Could you check a few things on this model? Use its own coordinates, in mm. Face numbers are marked on the shaded views. Coordinates: 2 decimals unless noted, no trailing zeros. Write each loop counter-clockwise with the first axis right and the second up, starting at its lowest first coordinate (ties: lowest second). Pieces come first, ordered by that corner, then holes. Notation, with made-up numbers: (-37.5, -33.5) - (-21.5, -33.5) arc R11 ccw to (-21.5, -22.5) - close; hole circle Ø4 at (76, 39). An arc over 180 degrees is marked (long way). Write item = value, one per line. Start each with the question number.
```python
from build123d import *

# Parameters (mm, degrees)
SKETCH1_R           = 4.064
SKETCH1_R_2         = 2.794
BOSS_EXTRUDE1_DEPTH = 3.302
SKETCH2_R           = 0.62500002
BOSS_EXTRUDE2_DEPTH = 1.87000007
SKETCH4_R           = 1.449999894
CUT_EXTRUDE1_DEPTH  = 21.9977138
SKETCH5_R           = 3.555000002
SKETCH5_R_2         = 2.819999948
BOSS_EXTRUDE3_DEPTH = 0.470000076


with BuildPart() as part:
    # Sketch1 → Boss-Extrude1 (new body)
    with BuildSketch(Plane(origin=(0, 0, 0), x_dir=(1, 0, 0), z_dir=(0, 1, 0))):
        with Locations(Location((0, 0, 0), (0, 0, 90))):
            Circle(SKETCH1_R)
        with Locations(Location((0, 0, 0), (0, 0, 90))):
            Circle(SKETCH1_R_2, mode=Mode.SUBTRACT)
    extrude(amount=BOSS_EXTRUDE1_DEPTH)

    # Sketch2 → Boss-Extrude2 (add)
    with BuildSketch(Plane(origin=(0, 3.302, 0), x_dir=(1, 0, 0), z_dir=(0, 1, 0))):
        with BuildLine():
            Line((3.184398134, 6.598095019), (1.973411671, 13.950499548))
            ThreePointArc((1.973411671, 13.950499548), (0, 15.24), (-1.973411671, 13.950499548))
            Line((-1.973411671, 13.950499548), (-3.184398134, 6.598095019))
            ThreePointArc((-3.184398134, 6.598095019), (-3.525092211, 6.105638812), (-4.121918835, 6.05681719))
            Line((-4.121918835, 6.05681719), (-11.094781168, 8.684274414))
            ThreePointArc((-11.094781168, 8.684274414), (-13.198227153, 7.620000001), (-13.068192838, 5.266225136))
            Line((-13.068192838, 5.266225136), (-7.306316969, 0.54127783))
            ThreePointArc((-7.306316969, 0.54127783), (-7.050184422, 1e-09), (-7.306316969, -0.541277828))
            Line((-7.306316969, -0.541277828), (-13.068192838, -5.266225133))
            ThreePointArc((-13.068192838, -5.266225133), (-13.198227153, -7.619999998), (-11.094781167, -8.684274411))
            Line((-11.094781167, -8.684274411), (-4.121918835, -6.056817187))
            ThreePointArc((-4.121918835, -6.056817187), (-3.525092211, -6.10563881), (-3.184398134, -6.598095016))
            Line((-3.184398134, -6.598095016), (-1.973411671, -13.950499545))
            ThreePointArc((-1.973411671, -13.950499545), (0, -15.239999997), (1.973411671, -13.950499545))
            Line((1.973411671, -13.950499545), (3.184398134, -6.598095017))
            ThreePointArc((3.184398134, -6.598095017), (3.525092211, -6.10563881), (4.121918835, -6.056817187))
            Line((4.121918835, -6.056817187), (11.094781168, -8.684274411))
            ThreePointArc((11.094781168, -8.684274411), (13.198227153, -7.619999998), (13.068192838, -5.266225133))
            Line((13.068192838, -5.266225133), (7.306316969, -0.541277828))
            ThreePointArc((7.306316969, -0.541277828), (7.050184422, 1e-09), (7.306316969, 0.54127783))
            Line((7.306316969, 0.54127783), (13.068192838, 5.266225136))
            ThreePointArc((13.068192838, 5.266225136), (13.198227153, 7.620000001), (11.094781167, 8.684274413))
            Line((11.094781167, 8.684274413), (4.121918835, 6.05681719))
            ThreePointArc((4.121918835, 6.05681719), (3.525092211, 6.105638812), (3.184398134, 6.598095019))
        make_face()
        with Locations(Location((0, -7.50046633, 0), (0, 0, 270))):
            Circle(SKETCH2_R, mode=Mode.SUBTRACT)
        with Locations(Location((0, -10.500466426, 0), (0, 0, 270))):
            Circle(SKETCH2_R, mode=Mode.SUBTRACT)
        with Locations(Location((0, -13.500466522, 0), (0, 0, 270))):
            Circle(SKETCH2_R, mode=Mode.SUBTRACT)
        with Locations(Location((-11.691746971, -6.750233261, 0), (0, 0, 270))):
            Circle(SKETCH2_R, mode=Mode.SUBTRACT)
        with Locations(Location((-9.093670677, -5.250233213, 0), (0, 0, 270))):
            Circle(SKETCH2_R, mode=Mode.SUBTRACT)
        with Locations(Location((-6.495594382, -3.750233165, 0), (0, 0, 270))):
            Circle(SKETCH2_R, mode=Mode.SUBTRACT)
        with Locations(Location((-11.691746971, 6.750233261, 0), (0, 0, 270))):
            Circle(SKETCH2_R, mode=Mode.SUBTRACT)
        with Locations(Location((-9.093670677, 5.250233213, 0), (0, 0, 270))):
            Circle(SKETCH2_R, mode=Mode.SUBTRACT)
        with Locations(Location((-6.495594382, 3.750233165, 0), (0, 0, 270))):
            Circle(SKETCH2_R, mode=Mode.SUBTRACT)
        with Locations(Location((0, 13.500466522, 0), (0, 0, 270))):
            Circle(SKETCH2_R, mode=Mode.SUBTRACT)
        with Locations(Location((0, 10.500466426, 0), (0, 0, 270))):
            Circle(SKETCH2_R, mode=Mode.SUBTRACT)
        with Locations(Location((0, 7.50046633, 0), (0, 0, 270))):
            Circle(SKETCH2_R, mode=Mode.SUBTRACT)
        with Locations(Location((11.691746971, 6.750233261, 0), (0, 0, 270))):
            Circle(SKETCH2_R, mode=Mode.SUBTRACT)
        with Locations(Location((9.093670677, 5.250233213, 0), (0, 0, 270))):
            Circle(SKETCH2_R, mode=Mode.SUBTRACT)
        with Locations(Location((6.495594382, 3.750233165, 0), (0, 0, 270))):
            Circle(SKETCH2_R, mode=Mode.SUBTRACT)
        with Locations(Location((11.691746971, -6.750233261, 0), (0, 0, 270))):
            Circle(SKETCH2_R, mode=Mode.SUBTRACT)
        with Locations(Location((9.093670677, -5.250233213, 0), (0, 0, 270))):
            Circle(SKETCH2_R, mode=Mode.SUBTRACT)
        with Locations(Location((6.495594382, -3.750233165, 0), (0, 0, 270))):
            Circle(SKETCH2_R, mode=Mode.SUBTRACT)
    extrude(amount=BOSS_EXTRUDE2_DEPTH)

    # Sketch4 → Cut-Extrude1 (cut, through all)
    with BuildSketch(Plane(origin=(0, 5.17200007, 0), x_dir=(1, 0, 0), z_dir=(0, 1, 0))):
        with Locations(Location((0, 0, 0), (0, 0, 270))):
            Circle(SKETCH4_R)
    extrude(amount=-CUT_EXTRUDE1_DEPTH, mode=Mode.SUBTRACT)

    # Sketch5 → Boss-Extrude3 (add)
    with BuildSketch(Plane(origin=(0, 5.17200007, 0), x_dir=(1, 0, 0), z_dir=(0, 1, 0))):
        with Locations(Location((0, 0, 0), (0, 0, 90))):
            Circle(SKETCH5_R)
        with Locations(Location((0, 0, 0), (0, 0, 270))):
            Circle(SKETCH5_R_2, mode=Mode.SUBTRACT)
    extrude(amount=BOSS_EXTRUDE3_DEPTH)


solid = part.part
```
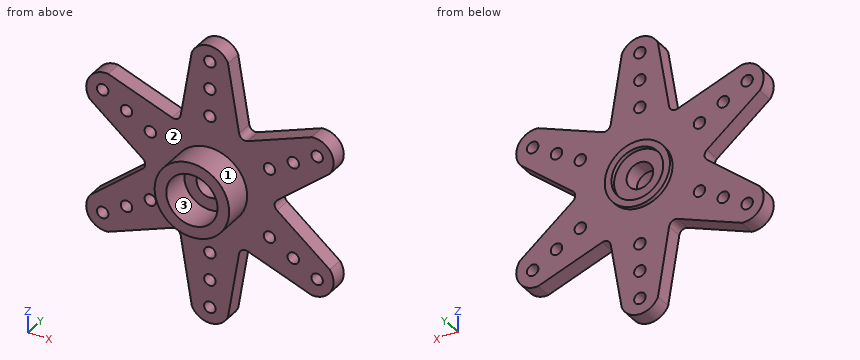
1) If I drill on probe 1 along X at (y, z) = (4.7, 0); probe 2 along X at (y, z) = (4.3, 5); probe 3 along Y at (x, z) = (-2, -8), over which ranges is the centre line in solid material (lowest first)? Write a range as [from, to].
2) For P1, Ø1.6, axis at x = 0, z = -7.5, coming from the -Y side; P2, Ø1.6, axis at x = 9.09, z = 5.25, coming from the +Y side; P3, Ø0.8, axis at x = 0, z = -10.5, coming from the +Y side, each with a flat end and sliding along its axis, tell me the tip position at first contact or that it passes through.
3) Suppose I cut it at A-A on z = 0. Please give me the cut outline in (x, y) (3 decimals), plus the area to 3 significant figures.
4) Suppose I cut it at B-B on x = -10.5. Please give me the cut outline in (y, z), plus the area to 3 significant figures.
5) Thinking about a two-plate mould opening in Z: for the marked faces 1, 2 and 3, which applies, +Z half, -Z half, draft (parallel to the pull), parting line (faces both ways), or undercut?
6) Suppose I cut it at D-D on x = 0. State how many separate pieces and enclosed holes the cut face has, plus the area to 3 significant figures.
7) Suppose I cut it at C-C on y = 1.2. Please give me the cut outline in (x, z).
Reply:
q1.probe_1 = [-7.05, -1.45], [1.45, 7.05]
q1.probe_2 = [-12.74, -9.67], [-8.52, 8.52], [9.67, 12.74]
q1.probe_3 = [3.3, 5.17]
q2.P1 = 3.3
q2.P2 = 5.17
q2.P3 = through
q3.outline = (-7.05, 3.302) - (-4.064, 3.302) - (-4.064, 0) - (-2.794, 0) - (-2.794, 3.302) - (-1.45, 3.302) - (-1.45, 5.172) - (-2.82, 5.172) - (-2.82, 5.642) - (-3.555, 5.642) - (-3.555, 5.172) - (-7.05, 5.172) - close; (1.45, 3.302) - (2.794, 3.302) - (2.794, 0) - (4.064, 0) - (4.064, 3.302) - (7.05, 3.302) - (7.05, 5.172) - (3.555, 5.172) - (3.555, 5.642) - (2.82, 5.642) - (2.82, 5.172) - (1.45, 5.172) - close
q3.area = 30.0 mm^2
q4.outline = (3.3, -8.46) - (5.17, -8.46) - (5.17, -3.16) - (3.3, -3.16) - close; (3.3, 3.16) - (5.17, 3.16) - (5.17, 8.46) - (3.3, 8.46) - close
q4.area = 19.8 mm^2
q5.face_1 = parting line
q5.face_2 = draft
q5.face_3 = undercut
q6.separate_pieces = 8
q6.enclosed_holes = 0
q6.area = 46.6 mm^2
q7.outline = circle Ø8.13 at (0, 0); hole circle Ø5.59 at (0, 0)
